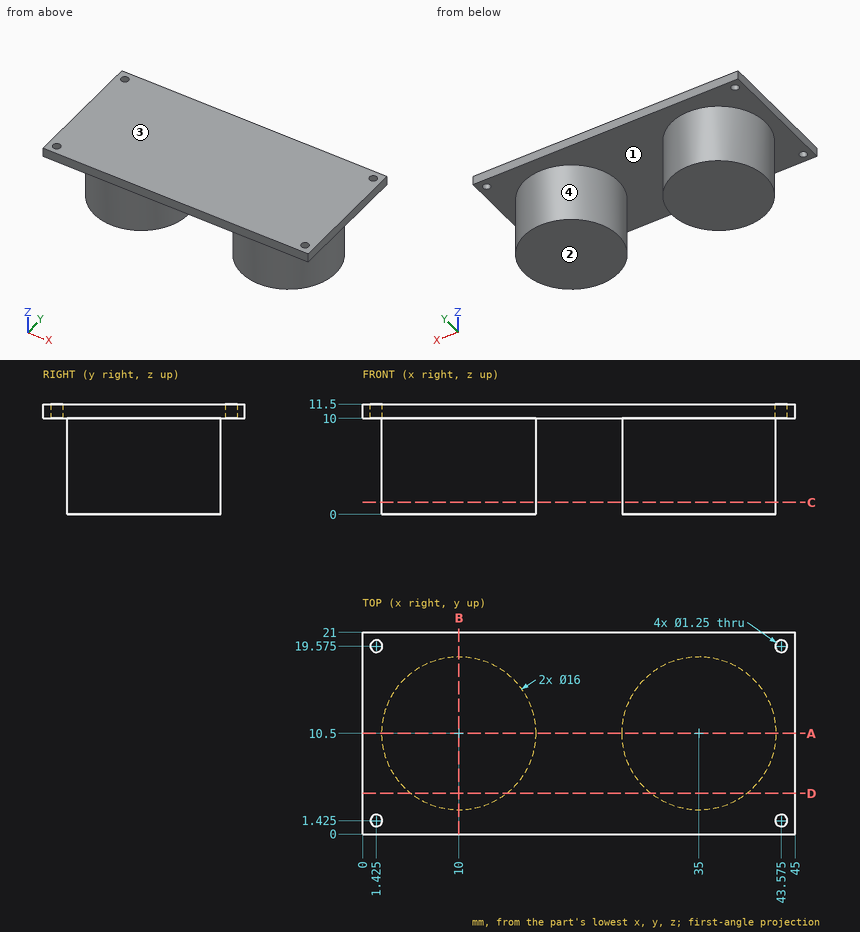
The drawing under review shows one solid part. Ordinate dimensions are in mm from its lowest x, y, z. A direction names the side the tool comes from. Give positions to 0.01 mm unless a question says otherwise; leave off trailing zeros. Loops run counter-clockwise (first coordinate to the right, second up) from the corner with the lowest first, then second, coordinate; pieces in that order, holes last. Notation, with made-up numbers: M 54,65 L 91,65 A24 cw 91,84 Z; hole C 21.25,27 d4. An arc over 180 degrees is marked long. One line per question, with ' | ' between items. Start each with the question number.
1. Insertion check: P1, Ø2, axis at x = 31, y = 13.5, coming from the -Z side; P2, Ø1, axis at x = 24, y = 16, coming from the -Z side. Each pin has a flat end and moves straight along its axis. Give the tip position at first contact, or say it passes through.
2. For the marked faces 1 and 2, list the 3-axis set-ups (+Z, -Z, +X, -X, +Y, -Y) from which the entire face can be reached by the end or side of a thin tool; tool diameter is ignored.
3. Add section C-C (z = 1.25). Write out the cut boundary in (x, y).
4. Add section B-B (x = 10). Write out the cut boundary in (y, z).
5. Add section A-A (y = 10.5). Write out the cut boundary in (x, z), plus the area to 4 significant figures.
6. Add section D-D (y = 4.25). Write out the cut boundary in (x, z), plus the area to 3 significant figures.
7. To check wall thickness, follow L1, parallel to X at y = 10.75, z = 3; L2, parallel to Z at x = 34, y = 18.75; L3, parallel to X at y = 4.5, z = 5.5. State the ranges of each line that lie inside material, in increasing order.
8. The part is to be moulded in two halves that separate along X. For the marked faces 3 and 4, say which applies: released by +X, released by -X, zero draft, split by the parting line, or undercut.
Worked out:
1) P1: stops at z = 0 | P2: stops at z = 10
2) face 1: -Z | face 2: -Z, +X, -X, +Y, -Y
3) outline: C 10,10.5 d16; C 35,10.5 d16
4) outline: M 0,10 L 2.5,10 L 2.5,0 L 18.5,0 L 18.5,10 L 21,10 L 21,11.5 L 0,11.5 Z
5) outline: M 0,10 L 2,10 L 2,0 L 18,0 L 18,10 L 27,10 L 27,0 L 43,0 L 43,10 L 45,10 L 45,11.5 L 0,11.5 Z | area: 387.5 mm²
6) outline: M 0,10 L 5.01,10 L 5.01,0 L 14.99,0 L 14.99,10 L 30.01,10 L 30.01,0 L 39.99,0 L 39.99,10 L 45,10 L 45,11.5 L 0,11.5 Z | area: 267 mm²
7) L1: x = 2 to 18, 27 to 43 | L2: z = 10 to 11.5 | L3: x = 4.71 to 15.29, 29.71 to 40.29
8) face 3: zero draft | face 4: undercut
